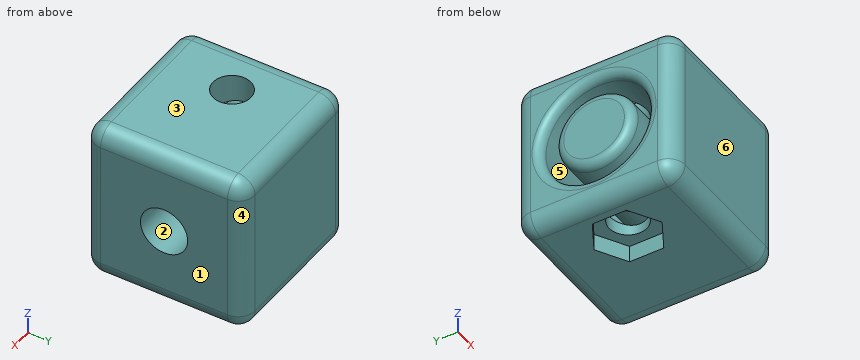
```python
from build123d import *

# Parameters (mm, degrees)
SKETCH1_W           = 19.05
SKETCH1_H           = 19.05
SKETCH1_R           = 6.35
BOSS_EXTRUDE1_DEPTH = 12.7
SKETCH3_W           = 19.05
SKETCH3_H           = 19.05
BOSS_EXTRUDE2_DEPTH = 6.35
SKETCH5_R           = 2.8
CUT_EXTRUDE1_DEPTH  = 7
SKETCH6_R           = 4.6
BOSS_EXTRUDE4_DEPTH = 12.7
CUT_EXTRUDE2_DEPTH  = 55
FILLET1_R           = 1
FILLET2_R           = 2
SKETCH9_R           = 2.25
CUT_EXTRUDE3_DEPTH  = 2


with BuildPart() as part:
    # Sketch1 → Boss-Extrude1 (new body)
    with BuildSketch(Plane(origin=(0, 0, 0), x_dir=(0, 0, -1), z_dir=(1, 0, 0))):
        Rectangle(SKETCH1_W, SKETCH1_H)
        Circle(SKETCH1_R, mode=Mode.SUBTRACT)
    extrude(amount=BOSS_EXTRUDE1_DEPTH)

    # Sketch3 → Boss-Extrude2 (add)
    with BuildSketch(Plane(origin=(12.7, 0, 0), x_dir=(0, 0, -1), z_dir=(1, 0, 0))):
        Rectangle(SKETCH3_W, SKETCH3_H)
    extrude(amount=BOSS_EXTRUDE2_DEPTH)

    # Sketch5 → Cut-Extrude1 (cut)
    with BuildSketch(Plane(origin=(19.05, 0, 0), x_dir=(0, 0, -1), z_dir=(1, 0, 0))):
        Circle(SKETCH5_R)
    extrude(amount=-CUT_EXTRUDE1_DEPTH, mode=Mode.SUBTRACT)

    # Sketch6 → Boss-Extrude4 (add)
    with BuildSketch(Plane.ZY.offset(-12.7)):
        Circle(SKETCH6_R)
    extrude(amount=BOSS_EXTRUDE4_DEPTH)

    # Sketch8 → Cut-Extrude2 (cut)
    with BuildSketch(Plane(origin=(0, 0, -9.525), x_dir=(-1, 0, 0), z_dir=(0, 0, -1))):
        with BuildLine():
            ThreePointArc((-4.1, 0), (-6.35, 2.25), (-8.6, 0))
            Line((-8.6, 0), (-4.1, 0))
        make_face()
        with BuildLine():
            Line((-4.1, 0), (-8.6, 0))
            ThreePointArc((-8.6, 0), (-6.35, -2.25), (-4.1, 0))
        make_face()
    extrude(amount=-CUT_EXTRUDE2_DEPTH, mode=Mode.SUBTRACT)

    # Fillet1
    fillet1_edges = [part.edges().sort_by_distance(p)[0] for p in [
        (0, 0, 6.35),
        (0, 0, -4.6),
    ]]
    fillet(fillet1_edges, radius=FILLET1_R)

    # Fillet2
    fillet2_edges = [part.edges().sort_by_distance(p)[0] for p in [
        (19.05, 9.525, 0),
        (19.05, 0, 9.525),
        (19.05, -9.525, 0),
        (19.05, 0, -9.525),
        (0, 9.525, 0),
        (0, 0, -9.525),
        (0, -9.525, 0),
        (0, 0, 9.525),
        (9.525, 9.525, 9.525),
        (9.525, 9.525, -9.525),
        (9.525, -9.525, -9.525),
        (9.525, -9.525, 9.525),
    ]]
    fillet(fillet2_edges, radius=FILLET2_R)

    # Sketch9 → Cut-Extrude3 (cut)
    with BuildSketch(Plane(origin=(0, 0, -9.525), x_dir=(-1, 0, 0), z_dir=(0, 0, -1))):
        Polygon((-9.85, 2.020725942), (-9.85, -2.020725942), (-6.35, -4.041451884), (-2.85, -2.020725942), (-2.85, 2.020725942), (-6.35, 4.041451884), align=None)
        with Locations((-6.35, 0)):
            Circle(SKETCH9_R, mode=Mode.SUBTRACT)
    extrude(amount=-CUT_EXTRUDE3_DEPTH, mode=Mode.SUBTRACT)


solid = part.part
```
Model file for the job. Use its own axes, mm. Face numbers are marked on the shaded views. A direction names the side the tool comes from. Give positions to 0.01 mm unless a question says otherwise; leave off trailing zeros. Write each loop counter-clockwise with the first axis right and the second up, starting at its lowest first coordinate (ties: lowest second). Pieces come first, ordered by that corner, then holes. Notation, with made-up numbers: M 87.5,87.5 L 97.5,87.5 A10 ccw 97.5,99.5 Z; hole C 22,-19 d10. An arc over 180 degrees is marked long. Use a Markdown table: item, result.
1) Pin check, flat tips, straight feed: pin 1 (0.6 mm diameter, centred on y = -0.5, z = -9, fed in from +X); pin 2 (6 mm diameter, centred on x = 6.35, y = 0, fed in from -Z) (3 decimals); pin 3 (3.5 mm diameter, centred on y = 0, z = 0, fed in from +X). Stop position of each tip, or through.
Responses:
| item | result |
|---|---|
| pin 1 | stops at x = 18.67 |
| pin 2 | stops at z = -7.525 |
| pin 3 | stops at x = 12.7 |
2) Cut at C-C (z = 0). List the corners of the cut face in (x, y) (3 decimals).
Responses:
| item | result |
|---|---|
| outline | M 0,-7.525 A2 ccw 2,-9.525 L 17.05,-9.525 A2 ccw 19.05,-7.525 L 19.05,-2.8 L 12.7,-2.8 L 12.7,2.8 L 19.05,2.8 L 19.05,7.525 A2 ccw 17.05,9.525 L 2,9.525 A2 ccw 0,7.525 L 0,7.35 A1 ccw 1,6.35 L 12.7,6.35 L 12.7,4.6 L 1,4.6 A1 ccw 0,3.6 L 0,-3.6 A1 ccw 1,-4.6 L 12.7,-4.6 L 12.7,-6.35 L 1,-6.35 A1 ccw 0,-7.35 Z; hole C 6.35,0 d4.5 |
3) Cut at B-B (x = 13.5). List the corners of the cut face in (y, z) (3 decimals).
Responses:
| item | result |
|---|---|
| outline | M -9.525,-7.525 A2 ccw -7.525,-9.525 L 7.525,-9.525 A2 ccw 9.525,-7.525 L 9.525,7.525 A2 ccw 7.525,9.525 L -7.525,9.525 A2 ccw -9.525,7.525 Z; hole C 0,0 d5.6 |
4) Drill centre lines: line 1 (Z direction, x = 9.25, y = 0) (3 decimals); line 2 (Y direction, x = 3.75, z = 0) (3 decimals). Where is each one in solid material? Low to high. Write a range as from..to.
Responses:
| item | result |
|---|---|
| line 1 | z = -7.525..-6.35, -4.6..4.6, 6.35..9.525 |
| line 2 | y = -9.525..-6.35, -4.6..4.6, 6.35..9.525 |
5) Cut at D-D (y = 0). Give the number of separate pieces and of enclosed holes in the cut face, and give its area (3 significant figures).
Responses:
| item | result |
|---|---|
| separate pieces | 4 |
| enclosed holes | 0 |
| area | 204 mm2 |
6) Pull direction Y, two halves, no side cores. Call the marked faces 3, 4, 5 and 6: +Y half, -Y half, draft (parallel to the pull), parting line (faces both ways), or undercut.
Responses:
| item | result |
|---|---|
| face 3 | draft |
| face 4 | +Y half |
| face 5 | undercut |
| face 6 | -Y half |
7) Tool access for the marked faces 1 and 2: list every direction of +Z, -Z, +X, -X, +Y, -Y with a clear straight run to the whole face (end or side of a thin tool).
Responses:
| item | result |
|---|---|
| face 1 | +Z, -Z, +X, +Y, -Y |
| face 2 | +X |
8) Cut at A-A (x = 10.25). List the corners of the cut face in (y, z) (3 decimals), and give its area (3 significant figures).
Responses:
| item | result |
|---|---|
| outline | M -9.525,-7.525 A2 ccw -7.525,-9.525 L 7.525,-9.525 A2 ccw 9.525,-7.525 L 9.525,7.525 A2 ccw 7.525,9.525 L -7.525,9.525 A2 ccw -9.525,7.525 Z; C 0,0 d9.2; hole C 0,0 d12.7 |
| area | 299 mm2 |
